Can you work these out from the model? Positions are in its coordinate system, mm. Face numbers are marked on the shaded views. A direction names the side the tool comes from. Give positions to 0.01 mm unless a question says otherwise; leave off trailing zeros. Order: outer loops, then holes, each group sorted by start corner. A loop starts at its lowest first (then second) coordinate and runs counter-clockwise, first axis right, second up. Notation, with made-up numbers: (-31.75, 22.5) - (17.25, 22.5) arc R13 cw to (17.25, 33.5) - close; hole circle Ø4 at (55, 80.5). An arc over 180 degrees is marked (long way). One line per question, with ' | ' between items.
```python
from build123d import *

# Parameters (mm, degrees)
F1_DEPTH  = 60.325
F3_DEPTH  = 41.3258
F5_DEPTH  = 19.05
F6_R      = 6.35
F7_DEPTH  = 22.353
F8_R      = 12.7
F9_DEPTH  = 60.326
F10_W     = 22.3266
F10_H     = 22.457045
F10_H_2   = 23.779094
F11_DEPTH = 57.151


with BuildPart() as f1:
    # F0 (on Right) → F1 (new body)
    with BuildSketch(Plane.YZ):
        with BuildLine():
            Line((108.502969, 0), (22.352, 0))
            ThreePointArc((22.352, 0), (0, 22.352), (-22.352, 0))
            ThreePointArc((-22.352, 0), (-15.805251, -15.805251), (0, -22.352))
            Line((0, -22.352), (194.2084, -22.352))
            Line((194.2084, -22.352), (194.2084, -7.874))
            ThreePointArc((194.2084, -7.874), (191.902159, -2.306241), (186.3344, 0))
            Line((186.3344, 0), (155.1686, 0))
            ThreePointArc((155.1686, 0), (151.576498, 1.487898), (150.0886, 5.08))
            Line((150.0886, 5.08), (150.0886, 29.718))
            ThreePointArc((150.0886, 29.718), (148.600702, 33.310102), (145.0086, 34.798))
            Line((145.0086, 34.798), (131.0386, 34.798))
            ThreePointArc((131.0386, 34.798), (123.482134, 14.995483), (108.502969, 0))
        make_face()
    extrude(amount=F1_DEPTH)

    # F2 (on face) → F3 (cut)
    with BuildSketch(Plane(origin=(0, 0, 0), x_dir=(0, -1, 0), z_dir=(-1, 0, 0))):
        with BuildLine():
            ThreePointArc((-150.0886, 5.08), (-151.576498, 1.487898), (-155.1686, 0))
            Line((-155.1686, 0), (-108.502969, 0))
            ThreePointArc((-108.502969, 0), (-123.482134, 14.995483), (-131.0386, 34.798))
            Line((-131.0386, 34.798), (-145.0086, 34.798))
            ThreePointArc((-145.0086, 34.798), (-148.600702, 33.310102), (-150.0886, 29.718))
            Line((-150.0886, 29.718), (-150.0886, 5.08))
        make_face()
    extrude(amount=-F3_DEPTH, mode=Mode.SUBTRACT)

    # F4 (on face) → F5 (cut)
    with BuildSketch(Plane.YZ.offset(60.325)):
        Polygon((108.502969, -22.352), (108.502969, 0), (85.852, 0), (91.8464, -22.352), align=None)
    extrude(amount=-F5_DEPTH, mode=Mode.SUBTRACT)

    # F6 (on face) → F7 (cut, through all)
    with BuildSketch(Plane.XY):
        with Locations((22.352, 147.4724)):
            Circle(F6_R)
    extrude(amount=-F7_DEPTH, mode=Mode.SUBTRACT)

    # F8 (on face) → F9 (cut, through all)
    with BuildSketch(Plane(origin=(0, 0, 0), x_dir=(0, -1, 0), z_dir=(-1, 0, 0))):
        Circle(F8_R)
    extrude(amount=-F9_DEPTH, mode=Mode.SUBTRACT)

    # F10 (on face) → F11 (cut, through all)
    with BuildSketch(Plane(origin=(0, 0, -22.352), x_dir=(1, 0, 0), z_dir=(0, 0, -1))):
        with Locations((30.1625, 11.228522)):
            Rectangle(F10_W, F10_H)
        with Locations((30.1625, -11.889547)):
            Rectangle(F10_W, F10_H_2)
    extrude(amount=-F11_DEPTH, mode=Mode.SUBTRACT)


solid = f1.part
```
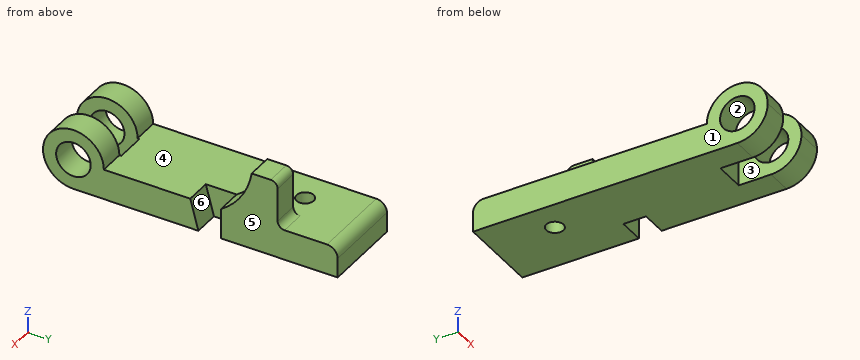
(1) Imagine slicing it at C-C (z = 9.5). List the corners of the cut face in (x, y) for me (3 decimals).
Answer below:
outline: (0, -20.233) - (18.999, -20.233) - (18.999, -8.429) - (0, -8.429) - close; (0, 8.429) - (18.999, 8.429) - (18.999, 20.233) - (0, 20.233) - close; (41.326, -20.233) - (60.325, -20.233) - (60.325, -8.429) - (41.326, -8.429) - close; (41.326, 8.429) - (60.325, 8.429) - (60.325, 20.233) - (41.326, 20.233) - close; (41.326, 119.371) - (60.325, 119.371) - (60.325, 150.089) - (41.326, 150.089) - close
(2) If I drill on line 1 (X direction, y = -4.5, z = 13) (3 decimals); line 2 (Z direction, x = 33, y = 124); line 3 (Y direction, x = 30, z = -13), over which ranges is the centre line in solid material (lowest first)?
Answer below:
line 1: 0 to 18.999, 41.326 to 60.325 | line 2: -22.35 to 0 | line 3: 23.78 to 194.21
(3) If we mould it in two halves opening along X, with no side actions, what happens to the marked faces 1, 2 and 3? For each: released by +X, released by -X, zero draft, split by the parting line, or undercut.
Answer below:
face 1: released by -X | face 2: zero draft | face 3: undercut
(4) Imagine slicing it at A-A (y = -4.5). List the corners of the cut face in (x, z) for me (3 decimals).
Answer below:
outline: (0, -21.894) - (18.999, -21.894) - (18.999, -11.876) - (0, -11.876) - close; (0, 11.876) - (18.999, 11.876) - (18.999, 21.894) - (0, 21.894) - close; (41.326, -21.894) - (60.325, -21.894) - (60.325, -11.876) - (41.326, -11.876) - close; (41.326, 11.876) - (60.325, 11.876) - (60.325, 21.894) - (41.326, 21.894) - close
(5) Will these pins go through, and if not, where does the flat tip stop? pin 1 (12 mm diameter, centred on x = 37, y = 150, fed in from +Z); pin 2 (15 mm diameter, centred on x = 49, z = 21.5, fed in from +Y); pin 3 (1 mm diameter, centred on x = 42.5, y = 45, fed in from +Z); pin 4 (1.5 mm diameter, centred on x = 40.5, y = 18, fed in from -Z).
Answer below:
pin 1: z = 34.73 | pin 2: y = 150.09 | pin 3: z = 0 | pin 4: through
(6) Imagine slicing it at D-D (y = 19). List the corners of the cut face in (x, z) for me (3 decimals), and give its area (3 significant figures).
Answer below:
outline: (0, -22.352) - (18.999, -22.352) - (18.999, 11.773) - (0, 11.773) - close; (41.326, -22.352) - (60.325, -22.352) - (60.325, 11.773) - (41.326, 11.773) - close | area: 1,300 mm^2
(7) On a 3-axis mill with a long thin cutter (end or side, diameter ignored), from which of +Z, -Z, +X, -X, +Y, -Y can I reach the whole of each face in a straight line? I mean the marked faces 4, 5 and 6. Say none if no direction works.
Answer below:
face 4: +Z, -X | face 5: +Z, -Z, +X, +Y, -Y | face 6: +Z, +X
(8) Imagine slicing it at B-B (x = 26.5). List the corners of the cut face in (y, z) for me, and give its area (3 significant figures).
Answer below:
outline: (23.78, -22.35) - (142.66, -22.35) - (142.66, 0) - (23.78, 0) - close; (152.28, -22.35) - (194.21, -22.35) - (194.21, -7.87) arc R7.87 ccw to (186.33, 0) - (152.28, 0) - close | area: 3,580 mm^2
